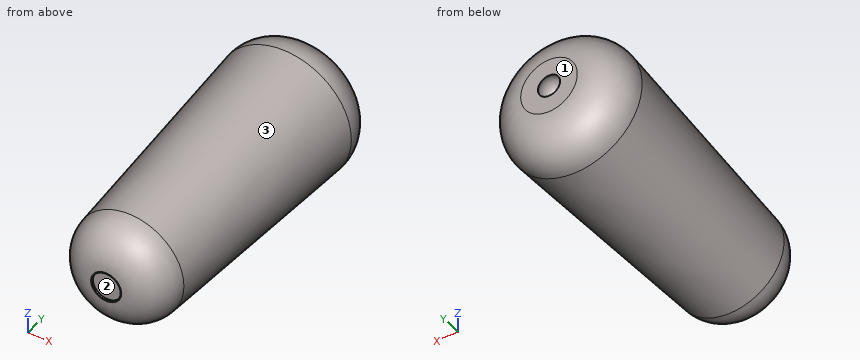
```python
from build123d import *

# Parameters (mm, degrees)
SKETCH1_R           = 90.957734813
SKETCH2_R           = 68.723621859
FILLET1_R           = 50.8
SKETCH5_R           = 19.05
BOSS_EXTRUDE1_DEPTH = 19.05
FILLET2_R           = 19.05
SKETCH6_R           = 19.05
CUT_EXTRUDE1_DEPTH  = 2.54


with BuildPart() as part:
    # Sketch1 → Loft1 section 0
    with BuildSketch(Plane(origin=(0, 0, 0), x_dir=(1, 0, 0), z_dir=(0, 1, 0))):
        Circle(SKETCH1_R)
    # Sketch2 → Loft1 section 1
    with BuildSketch(Plane(origin=(0, -415, 0), x_dir=(-1, 0, 0), z_dir=(0, 1, 0))):
        Circle(SKETCH2_R)
    loft()

    # Fillet1
    fillet1_edges = [part.edges().sort_by_distance(p)[0] for p in [
        (-68.723621859, -415, 0),
        (-90.957734813, 0, 0),
    ]]
    fillet(fillet1_edges, radius=FILLET1_R)


with BuildPart() as body_2:
    # Sketch5 → Boss-Extrude1 (new, symmetric)
    with BuildSketch(Plane.XY):
        with Locations(Location((0, -12.241562165, 0), (0, 0, 180))):
            Circle(SKETCH5_R)
    extrude(amount=BOSS_EXTRUDE1_DEPTH, both=True)

    # Fillet2
    fillet2_edges = [body_2.edges().sort_by_distance(p)[0] for p in [
        (19.05, -12.241562165, -19.05),
        (19.05, -12.241562165, 19.05),
    ]]
    fillet(fillet2_edges, radius=FILLET2_R - 0.0001)  # a hair under: the kernel refuses the full size


with BuildPart() as part_1:
    add(part.part)

    # Combine1: cut body 2
    add(body_2.part, mode=Mode.SUBTRACT)

    # Sketch6 → Cut-Extrude1 (cut)
    with BuildSketch(Plane.XZ.offset(415)):
        with Locations(Location((0, 0, 0), (0, 0, 270))):
            Circle(SKETCH6_R)
    extrude(amount=-CUT_EXTRUDE1_DEPTH, mode=Mode.SUBTRACT)


solid = part_1.part
```
Work out the finished part from the listing and answer in its coordinate system (mm). Face numbers are marked on the shaded views. Give positions to 0.01 mm unless a question says otherwise; leave off trailing zeros. Write each loop counter-clockwise with the first axis right and the second up, starting at its lowest first coordinate (ties: lowest second). Pieces come first, ordered by that corner, then holes.
(1) The part is cut by section B-B on y = -253.5. Write down the section's boundary in (x, z).
Final values:
outline: circle Ø154.75 at (0, 0)
(2) The part is cut by section A-A on y = -186.5. Write down the section's boundary in (x, z), plus the area to 3 significant figures.
Final values:
outline: circle Ø161.93 at (0, 0)
area: 20,600 mm2
(3) The mould has two halves that part along X. Classify the marked faces 1, 2 and 3: pulls with the +X half, pulls with the -X half, needs draft (parallel to the pull), parting line crosses it, or undercut.
Final values:
face 1: needs draft
face 2: undercut
face 3: parting line crosses it
(4) Straight lines are drawn through the part: line 1 (Y direction, x = 0, z = 0); line 2 (Y direction, x = -6.5, z = -22); line 3 (X direction, y = -97.5, z = -7). For each, find the intervals that lie inside material, in ascending order.
Final values:
line 1: y = -412.46 to -31.29
line 2: y = -414.94 to 0
line 3: x = -85.45 to 85.45
(5) Flat-ended cylindrical pins translate along their axes: pin 1 Ø6 at (x, z) = (51.5, -15.5) entering from +Y; pin 2 Ø23 at (x, z) = (0, 0) entering from -Y; pin 3 Ø4 at (x, z) = (-45, 13) entering from +Y. Find the tip coordinate at first contact, or state that the pin passes through.
Final values:
pin 1: stops at y = -1.8
pin 2: stops at y = -412.46
pin 3: stops at y = -0.55
